Design review of the part shown in the three views and the two pictorial views. Dimensions are in mm from the part's minimum x, y and z. Give positions to 0.01 mm unless a question says otherwise; leave off trailing zeros. Order: outer loops, then holes, each group sorted by start corner. A loop starts at its lowest first (then second) coordinate and runs counter-clockwise, first axis right, second up.
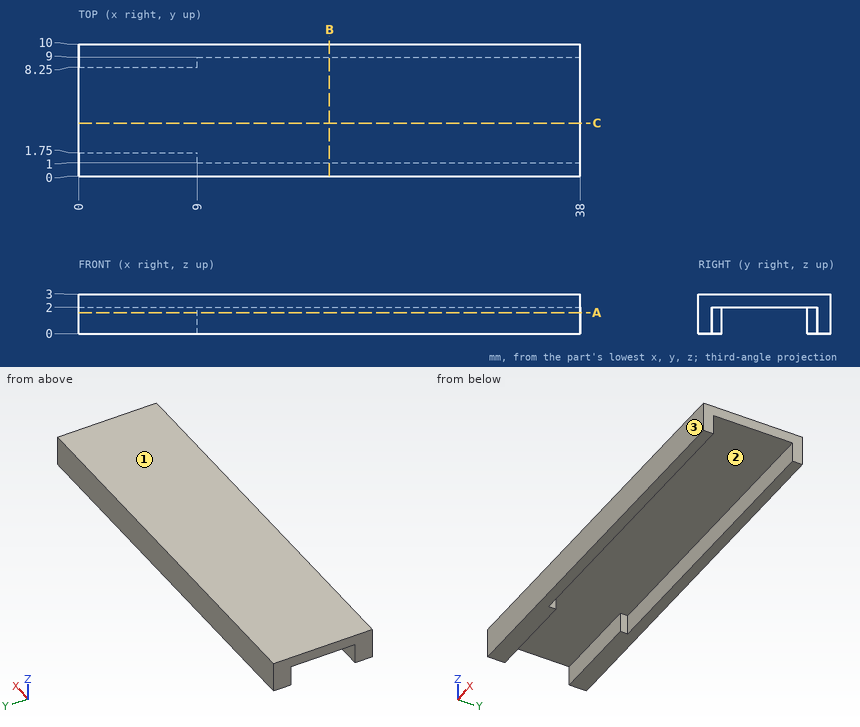
Item 1: Take a section at C-C (y = 4). Give the boundary of the cut face in (x, z).
Values found:
outline: (0, 2) - (38, 2) - (38, 3) - (0, 3) - close
Item 2: For line 1 (Y direction, x = 20, z = 1.4); line 2 (Y direction, x = 2, z = 1.2); line 3 (Z direction, x = 17, y = 7), list the stretches that pass through material, from the lowest coordinate up.
Values found:
line 1: y = 0 to 1, 9 to 10
line 2: y = 0 to 1.75, 8.25 to 10
line 3: z = 2 to 3
Item 3: Take a section at B-B (x = 19). Give the boundary of the cut face in (y, z).
Values found:
outline: (0, 0) - (1, 0) - (1, 2) - (9, 2) - (9, 0) - (10, 0) - (10, 3) - (0, 3) - close
Item 4: Take a section at A-A (z = 1.6). Give the boundary of the cut face in (x, y).
Values found:
outline: (0, 0) - (38, 0) - (38, 1) - (9, 1) - (9, 1.75) - (0, 1.75) - close; (0, 8.25) - (9, 8.25) - (9, 9) - (38, 9) - (38, 10) - (0, 10) - close
Item 5: Clearance check with a flat-ended pin moving along its axis: pin 1 Ø1 at (x, y) = (14, 3.5) entering from -Z. State where the tip first meets the part, or that it passes through.
Values found:
pin 1: stops at z = 2
Item 6: Draft analysis for pull direction Y (two halves, no side actions). For the marked faces 1, 2 and 3, state which applies: released by +Y, released by -Y, zero draft, split by the parting line, or undercut.
Values found:
face 1: zero draft
face 2: undercut
face 3: released by -Y
